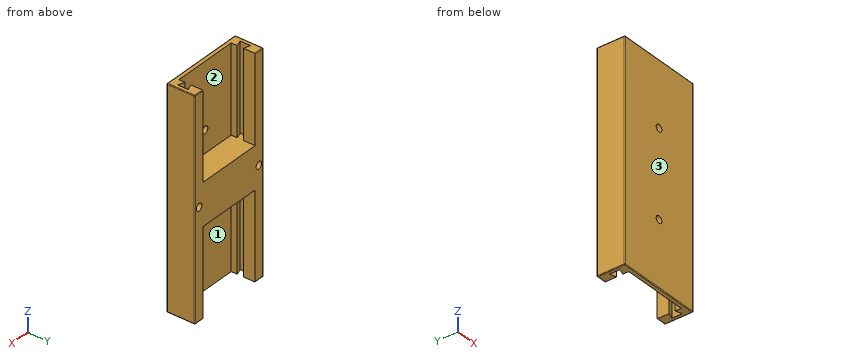
Autodesk Inventor part; units mm, degrees
ref_plane "YZ Plane" through (0, 0, 0) normal (1, 0, 0) x (0, 1, 0)
ref_plane "XZ Plane" through (0, 0, 0) normal (0, 1, 0) x (-1, 0, 0)
ref_plane "XY Plane" through (0, 0, 0) normal (0, 0, 1) x (1, 0, 0)
sketch "Sketch1" plane through (0, 0, 0) normal (0, 0, 1) x (1, 0, 0)
  line L0 (0, 0) -> (40, 0)
  line L1 (40, 0) -> (40, 13)
  line L2 (40, 13) -> (0, 13)
  line L3 (0, 13) -> (0, 0)
  dimension "d0" = 40
  dimension "d1" = 13
extrude "Extrusion1" add sketch "Sketch1" against normal blind 100
sketch "Sketch2" plane through (0, 0, 0) normal (0, 0, 1) x (1, 0, 0)
  line L0 (4.7, 1.898) -> (35.3, 1.898)
  line L1 (38.3, 8.5152) -> (38.3, 3.6828)
  line L2 (1.7, 8.5152) -> (1.7, 3.6828)
  line L3 (35.3, 7.5152) -> (38.3, 8.5152)
  line L4 (35.3, 7.5152) -> (35.3, 13)
  line L5 (35.3, 1.898) -> (35.3, 4.6828)
  line L6 (38.3, 3.6828) -> (35.3, 4.6828)
  line L7 (4.7, 7.5152) -> (1.7, 8.5152)
  line L8 (4.7, 13) -> (4.7, 7.5152)
  line L9 (4.7, 4.6828) -> (4.7, 1.898)
  line L10 (1.7, 3.6828) -> (4.7, 4.6828)
  line L11 (4.7, 13) -> (35.3, 13)
  point P0 (0, 13)
  point P1 (40, 13)
extrude "Extrusion2" cut sketch "Sketch2" against normal blind 40.3
sketch "Sketch3" plane through (0, 0, -100) normal (0, 0, -1) x (-1, 0, 0)
  line L0 (-35.3, 1.898) -> (-4.7, 1.898)
  line L1 (-1.7, 8.5152) -> (-1.7, 3.6828)
  line L2 (-38.3, 8.5152) -> (-38.3, 3.6828)
  line L3 (-4.7, 7.5152) -> (-1.7, 8.5152)
  line L4 (-4.7, 7.5152) -> (-4.7, 13)
  line L5 (-4.7, 1.898) -> (-4.7, 4.6828)
  line L6 (-1.7, 3.6828) -> (-4.7, 4.6828)
  line L7 (-35.3, 7.5152) -> (-38.3, 8.5152)
  line L8 (-35.3, 13) -> (-35.3, 7.5152)
  line L9 (-35.3, 4.6828) -> (-35.3, 1.898)
  line L10 (-38.3, 3.6828) -> (-35.3, 4.6828)
  line L11 (-35.3, 13) -> (-4.7, 13)
  point P0 (-40, 13)
  point P1 (0, 13)
extrude "Extrusion3" cut sketch "Sketch3" against normal blind 40.3
sketch "Sketch5" plane through (4.7, 1.898, 0) normal (0, 1, 0) x (1, 0, 0)
  circle A0 centre (15.3, 30) radius 1.65
  line L0 (35.3, 0) -> (35.3, 100)
  circle A1 centre (15.3, 70) radius 1.65
  point P0 (-4.7, 0)
extrude "Extrusion5" cut sketch "Sketch5" against normal blind 5
fillet "Fillet1" radius 0.3 14 edges at (2.35, 13, -100) (37.65, 13, -100) (0, 6.5, -100) (0, 13, -50) (0, 0, -50) (20, 0, -100) (40, 6.5, -100) (0, 6.5, 0) (40, 13, -50) (40, 0, -50) (20, 0, 0) (40, 6.5, 0) (2.35, 13, 0) (37.65, 13, 0)
sketch "Sketch6" plane through (4.7, 13, -40.3) normal (0, 1, 0) x (1, 0, 0)
  line L0 (-4.4, -40) -> (-4.4, 59.4)
  line L1 (-4.7, 59.4) -> (-4.7, -40)
  line L2 (35.3, -40) -> (35.3, 59.4)
  circle A0 centre (32.8, 9.7) radius 1.65
  circle A1 centre (-2.2, 9.7) radius 1.65
  point P0 (-4.7, -40.3)
  dimension "d29" = 3.3
  dimension "d30" = 3.3
extrude "Extrusion6" cut sketch "Sketch6" against normal blind 10
properties part number "centralBodyThick"
CAD build for the part. Positions are in the model's coordinates, mm. Face numbers are marked on the shaded views. A direction names the side the tool comes from. Round coordinates to 2 decimals unless told otherwise and drop trailing zeros. Loops run counter-clockwise (first coordinate to the right, second up) from the corner with the lowest first, then second, coordinate; pieces in that order, holes last. Notation, with made-up numbers: (-26.5, -7.5) - (-8.5, -7.5) arc R8 cw to (-8.5, 5.5) - close; hole circle Ø3 at (-24.75, 28). An arc over 180 degrees is marked (long way). Return JSON: item names as keys, results as strings. Group by question number.
Q1. Band-saw the part on B-B on x = 20. Give the cut face in (y, z), plus the area to 3 significant figures.
Q2. Flat gauge pins, fed straight in: pin 1 Ø1 at (x, y) = (17, 10.5) entering from +Z; pin 2 Ø4 at (x, z) = (20, -70) entering from +Y. Where does each tip first touch, or does it go through?
Q3. Drill centre lines: line 1 along Z through (x, y) = (20, 0.95); line 2 along X through (y, z) = (5.75, -50); line 3 along X through (y, z) = (0.5, -30). Where is each one in solid material? Low to high. Write a range as [from, to].
Q4. Band-saw the part on C-C on y = 10.25. Give the cut face in (x, z).
Q5. Band-saw the part on A-A on z = -70. Give the cut face in (x, y).
Q6. Tool access for the marked faces 1, 2 and 3: list every direction of +Z, -Z, +X, -X, +Y, -Y with a clear straight run to the whole face (end or side of a thin tool).
Q7. Band-saw the part on D-D on z = -50. Give the cut face in (x, y), plus the area to 3 significant figures.
Solutions:
{
 "1": {"outline": "(0, -99.7) arc R0.3 ccw to (0.3, -100) - (1.9, -100) - (1.9, -71.65) - (0, -71.65) - close; (0, -68.35) - (1.9, -68.35) - (1.9, -59.7) - (13, -59.7) - (13, -40.3) - (1.9, -40.3) - (1.9, -31.65) - (0, -31.65) - close; (0, -28.35) - (1.9, -28.35) - (1.9, 0) - (0.3, 0) arc R0.3 ccw to (0, -0.3) - close", "area": "393 mm^2"},
 "2": {"pin 1": "stops at z = -40.3", "pin 2": "stops at y = 1.9"},
 "3": {"line 1": "z = [-100, -71.65], [-68.35, -31.65], [-28.35, 0]", "line 2": "x = [0, 0.85], [4.15, 35.85], [39.15, 40]", "line 3": "x = [0, 18.35], [21.65, 40]"},
 "4": {"outline": "(0, -99.7) arc R0.3 ccw to (0.3, -100) - (4.7, -100) - (4.7, -59.7) - (35.3, -59.7) - (35.3, -100) - (39.7, -100) arc R0.3 ccw to (40, -99.7) - (40, -0.3) arc R0.3 ccw to (39.7, 0) - (35.3, 0) - (35.3, -40.3) - (4.7, -40.3) - (4.7, 0) - (0.3, 0) arc R0.3 ccw to (0, -0.3) - close; hole circle Ø3.3 at (2.5, -50); hole circle Ø3.3 at (37.5, -50)"},
 "5": {"outline": "(0, 0.3) arc R0.3 ccw to (0.3, 0) - (18.35, 0) - (18.35, 1.9) - (4.7, 1.9) - (4.7, 4.68) - (1.7, 3.68) - (1.7, 8.52) - (4.7, 7.52) - (4.7, 13) - (0.3, 13) arc R0.3 ccw to (0, 12.7) - close; (21.65, 0) - (39.7, 0) arc R0.3 ccw to (40, 0.3) - (40, 12.7) arc R0.3 ccw to (39.7, 13) - (35.3, 13) - (35.3, 7.52) - (38.3, 8.52) - (38.3, 3.68) - (35.3, 4.68) - (35.3, 1.9) - (21.65, 1.9) - close"},
 "6": {"face 1": "-Z, +Y", "face 2": "+Z, +Y", "face 3": "+Z, -Z, +X, -X, -Y"},
 "7": {"outline": "(0, 0.3) arc R0.3 ccw to (0.3, 0) - (39.7, 0) arc R0.3 ccw to (40, 0.3) - (40, 12.7) arc R0.3 ccw to (39.7, 13) - (39.15, 13) - (39.15, 3) - (35.85, 3) - (35.85, 13) - (4.15, 13) - (4.15, 3) - (0.85, 3) - (0.85, 13) - (0.3, 13) arc R0.3 ccw to (0, 12.7) - close", "area": "454 mm^2"}
}
